from build123d import *

# Parameters (mm, degrees)
SKETCH1_W           = 70
SKETCH1_H           = 70
BOSS_EXTRUDE1_DEPTH = 20
BOSS_EXTRUDE3_DEPTH = 15


with BuildPart() as part:
    # Sketch1 → Boss-Extrude1 (new body)
    with BuildSketch(Plane(origin=(0, 0, 0), x_dir=(1, 0, 0), z_dir=(0, 1, 0))):
        with Locations((-35, -35)):
            Rectangle(SKETCH1_W, SKETCH1_H)
    extrude(amount=BOSS_EXTRUDE1_DEPTH)

    # Sketch2 → Boss-Extrude3 (add)
    with BuildSketch(Plane(origin=(0, 20, 0), x_dir=(1, 0, 0), z_dir=(0, 1, 0))):
        Polygon((-55, -22), (-53.2, -22), (-53.2, -19.5), (-51.7, -19.5), (-49.08370491, -22.11629509), (-49.08370491, -27.61629509), (-51.7, -30.232590181), (-53.2, -30.232590181), (-53.2, -28.032590181), (-55, -28.032590181), align=None)
        Polygon((-16.8, -28.032590181), (-15, -28.032590181), (-15, -22), (-16.8, -22), (-16.8, -19.5), (-18.3, -19.5), (-20.91629509, -22.11629509), (-20.91629509, -27.61629509), (-18.3, -30.232590181), (-16.8, -30.232590181), align=None)
        Polygon((-53.2, -41.967409819), (-55, -41.967409819), (-55, -48), (-53.2, -48), (-53.2, -50.5), (-51.7, -50.5), (-49.08370491, -47.88370491), (-49.08370491, -42.38370491), (-51.7, -39.767409819), (-53.2, -39.767409819), align=None)
        Polygon((-16.8, -39.767409819), (-16.8, -41.967409819), (-15, -41.967409819), (-15, -48), (-16.8, -48), (-16.8, -50.5), (-18.3, -50.5), (-20.91629509, -47.88370491), (-20.91629509, -42.38370491), (-18.3, -39.767409819), align=None)
    extrude(amount=BOSS_EXTRUDE3_DEPTH)


solid = part.part
The listing builds one solid part. Answer for the finished solid, in the listing's coordinates (mm). A direction names the side the tool comes from. Coordinates: 2 decimals unless noted, no trailing zeros. Write each loop counter-clockwise with the first axis right and the second up, starting at its lowest first coordinate (ties: lowest second). Pieces come first, ordered by that corner, then holes. Notation, with made-up numbers: (29.5, -19) - (63.5, -19) arc R20 ccw to (63.5, -7) - close; hole circle Ø10 at (-39.75, 6.25). An arc over 180 degrees is marked (long way). Put each result on its own line as item: value.
1. The part is cut by section D-D on z = 33.5. Give the vertices of the cut face in (x, y).
Answer sheet:
outline: (-70, 0) - (0, 0) - (0, 20) - (-70, 20) - close
2. The part is cut by section B-B on y = 32.5. State how many separate pieces and enclosed holes the cut face has, plus the area to 3 significant figures.
Answer sheet:
separate pieces: 4
enclosed holes: 0
area: 193 mm^2
3. The part is cut by section C-C on x = -14. Give the vertices of the cut face in (y, z), plus the area to 3 significant figures.
Answer sheet:
outline: (0, 0) - (20, 0) - (20, 70) - (0, 70) - close
area: 1,400 mm^2
4. The part is cut by section A-A on z = 24. Give the vertices of the cut face in (x, y), plus the area to 3 significant figures.
Answer sheet:
outline: (-70, 0) - (0, 0) - (0, 20) - (-15, 20) - (-15, 35) - (-20.92, 35) - (-20.92, 20) - (-49.08, 20) - (-49.08, 35) - (-55, 35) - (-55, 20) - (-70, 20) - close
area: 1,580 mm^2
5. Find the intervals of material crossed by line 1 along Y through (x, z) = (-59.5, 29), in increasing order. Write a range as from..to.
Answer sheet:
line 1: y = 0..20
6. Determine the mould class of faces 5 (the face through (-54, 27, 22)), 6 (the face through (-15, 27, 25)), 7 (the face through (-50.4, 27.4, 20.8)) for opening direction X: pulls with the +X half, pulls with the -X half, needs draft (parallel to the pull), parting line crosses it, or undercut.
Answer sheet:
face 5: needs draft
face 6: pulls with the +X half
face 7: undercut
7. A tool of negligible diameter and unlimited length cuts with its end or side. For faces 1 (the face through (-16, 27, 28.033)), 2 (the face through (-20.916, 27, 45)), 3 (the face through (-16.8, 27, 49)), 4 (the face through (-19.6, 27.4, 49.2)), from which of +Z, -Z, +X, -X, +Y, -Y can it reach the whole face along a straight path? Write none if from no direction.
Answer sheet:
face 1: +X, +Y
face 2: +Z, -Z, +Y
face 3: +Z, +X, +Y
face 4: +Z, +Y
8. Flat-ended cylindrical pins translate along their axes: pin 1 Ø0.5 at (x, y) = (-15.5, 25) entering from -Z; pin 2 Ø1.6 at (y, z) = (29.5, 25.5) entering from +X; pin 3 Ø0.8 at (x, y) = (-17.5, 30) entering from -Z; pin 4 Ø1.5 at (y, z) = (30, 38.5) entering from +X. Find the tip coordinate at first contact, or state that the pin passes through.
Answer sheet:
pin 1: stops at z = 22
pin 2: stops at x = -15
pin 3: stops at z = 19.5
pin 4: passes through
